The drawing under review shows one solid part. Ordinate dimensions are in mm from its lowest x, y, z. A direction names the side the tool comes from. Give positions to 0.01 mm unless a question says otherwise; leave off trailing zeros. Write each loop counter-clockwise with the first axis right and the second up, starting at its lowest first coordinate (ties: lowest second). Pieces come first, ordered by that corner, then holes. Notation, with made-up numbers: M -37,-12 L 16,-12 A17 ccw 16,20 Z; hole C 2,64 d3. An arc over 180 degrees is marked long. One line per item, written item: value. Start each with the question number.
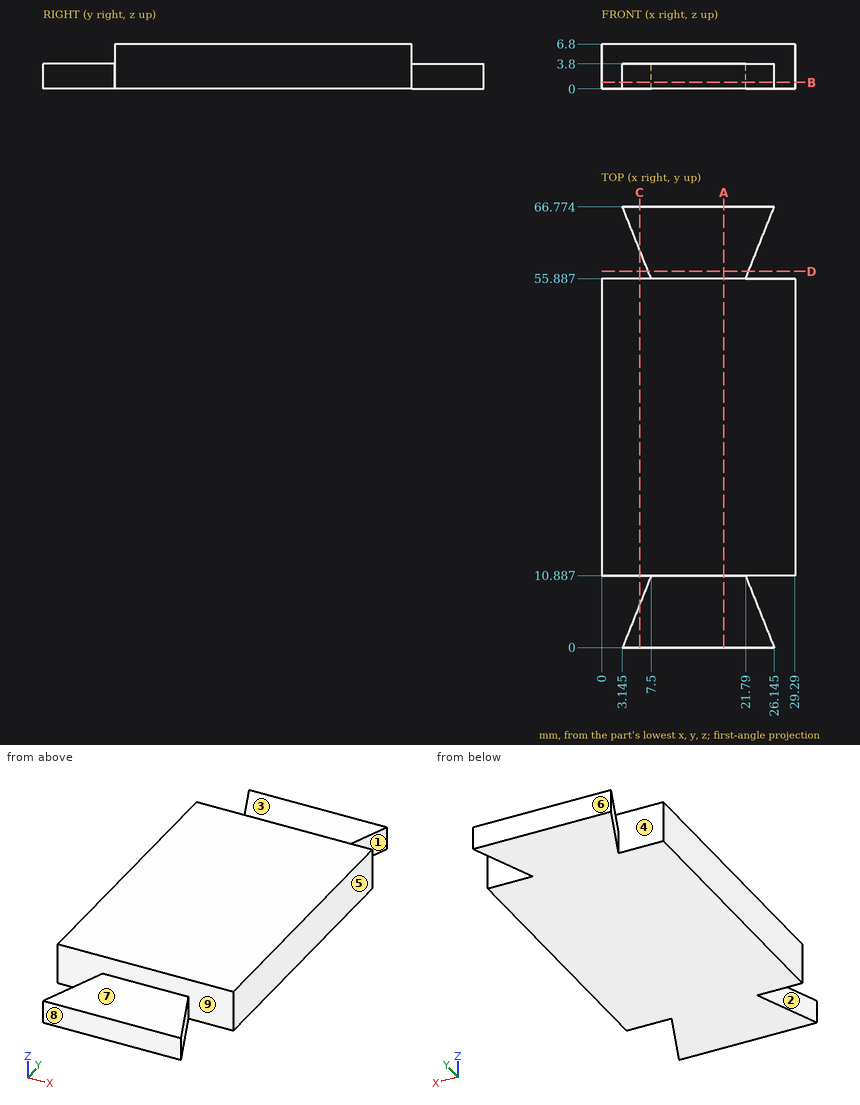
Q1. Take a section at A-A, the plane x = 18.5. Give the boundary of the cut face in (y, z), then the cut area to 3 significant figures.
Q2. For P1, Ø3.5, axis at x = 17.5, y = 4, coming from the +Z side, flat-tipped, find the tip position at first contact; note if it passes through.
Q3. Wall thickness on line 1 (Y direction, x = 24.5, z = 3.25) (1 decimal); line 2 (Y direction, x = 22, z = 2.5) (1 decimal); line 3 (Y direction, x = 22, z = 5.25): over which ranges is each line inside the solid? List them lowest first. Write a range as from..to.
Q4. Take a section at C-C, the plane x = 5.75. Give the boundary of the cut face in (y, z).
Q5. Take a section at B-B, the plane z = 1. Give the boundary of the cut face in (x, y) (1 decimal), then the cut area to 3 significant figures.
Q6. Machinability: for the marked faces 1, 2, 3, 4 and 5, which of the approach directions +Z, -Z, +X, -X, +Y, -Y give a long, thin tool a straight path to every point of the face, cutting with its end or side? Answer none if there is none.
Q7. Take a section at D-D, the plane y = 57. Give the boundary of the cut face in (x, z) (1 decimal).
Q8. The part is to be moulded in two halves that separate along Y. For the marked faces 6, 7, 8 and 9, say which applies: pulls with the +Y half, pulls with the -Y half, needs draft (parallel to the pull), parting line crosses it, or undercut.
Results list:
1. outline: M 0,0 L 66.77,0 L 66.77,3.8 L 55.89,3.8 L 55.89,6.8 L 10.89,6.8 L 10.89,3.8 L 0,3.8 Z
1. area: 389 mm^2
2. P1: stops at z = 3.8
3. line 1: y = 0..4.1, 10.9..55.9, 62.7..66.8
3. line 2: y = 0..10.4, 10.9..55.9, 56.4..66.8
3. line 3: y = 10.89..55.89
4. outline: M 0,0 L 6.51,0 L 6.51,3.8 L 0,3.8 Z; M 10.89,0 L 55.89,0 L 55.89,6.8 L 10.89,6.8 Z; M 60.26,0 L 66.77,0 L 66.77,3.8 L 60.26,3.8 Z
5. outline: M 0,10.9 L 7.5,10.9 L 3.1,0 L 26.1,0 L 21.8,10.9 L 29.3,10.9 L 29.3,55.9 L 21.8,55.9 L 26.1,66.8 L 3.1,66.8 L 7.5,55.9 L 0,55.9 Z
5. area: 1,720 mm^2
6. face 1: +Z, -Z, +X
6. face 2: +Z, -Z, -X
6. face 3: +Z, +X, -X, +Y
6. face 4: +Z
6. face 5: +Z, -Z, +X, +Y, -Y
7. outline: M 7.1,0 L 22.2,0 L 22.2,3.8 L 7.1,3.8 Z
8. face 6: pulls with the +Y half
8. face 7: needs draft
8. face 8: pulls with the -Y half
8. face 9: undercut
